from build123d import *

# Parameters (mm, degrees)
BOSS_EXTRUDE1_DEPTH = 70
SKETCH2_R           = 5
CUT_EXTRUDE1_DEPTH  = 816
SKETCH3_R           = 10
CUT_EXTRUDE2_DEPTH  = 143
FILLET1_R           = 4


with BuildPart() as part:
    # Sketch1 → Boss-Extrude1 (new body)
    with BuildSketch(Plane.XY):
        with BuildLine():
            Line((-110, 0), (90, 0))
            ThreePointArc((90, 0), (266.776695297, -73.223304703), (340, -250))
            Line((340, -250), (340, -350))
            Line((340, -350), (350, -350))
            Line((350, -350), (350, -240))
            ThreePointArc((350, -240), (276.776695297, -63.223304703), (100, 10))
            Line((100, 10), (-120, 10))
            ThreePointArc((-120, 10), (-296.776695297, -63.223304703), (-370, -240))
            Line((-370, -240), (-370, -350))
            Line((-370, -350), (-360, -350))
            Line((-360, -350), (-360, -250))
            ThreePointArc((-360, -250), (-286.776695297, -73.223304703), (-110, 0))
        make_face()
    extrude(amount=BOSS_EXTRUDE1_DEPTH)

    # Sketch2 → Cut-Extrude1 (cut)
    with BuildSketch(Plane(origin=(350, 0, 0), x_dir=(0, 0, -1), z_dir=(1, 0, 0))):
        with Locations((-36.389856075, -325)):
            Circle(SKETCH2_R)
    extrude(amount=-CUT_EXTRUDE1_DEPTH, mode=Mode.SUBTRACT)

    # Sketch3 → Cut-Extrude2 (cut)
    with BuildSketch(Plane(origin=(0, 10, 0), x_dir=(1, 0, 0), z_dir=(0, 1, 0))):
        with Locations((-65, -35)):
            Circle(SKETCH3_R)
        with Locations((-10, -35)):
            Circle(SKETCH3_R)
        with Locations((45, -35)):
            Circle(SKETCH3_R)
    extrude(amount=-CUT_EXTRUDE2_DEPTH, mode=Mode.SUBTRACT)

    # Fillet1
    fillet1_edges = [part.edges().sort_by_distance(p)[0] for p in [
        (-296.776695297, -63.223304703, 70),
        (350, -295, 0),
        (345, -350, 0),
        (340, -300, 0),
        (266.776695297, -73.223304703, 0),
        (-10, 0, 0),
        (-286.776695297, -73.223304703, 0),
        (-370, -295, 70),
        (-360, -300, 0),
        (-365, -350, 0),
        (-370, -295, 0),
        (-296.776695297, -63.223304703, 0),
        (-10, 10, 0),
        (276.776695297, -63.223304703, 0),
        (-365, -350, 70),
        (-360, -300, 70),
        (-286.776695297, -73.223304703, 70),
        (-10, 0, 70),
        (266.776695297, -73.223304703, 70),
        (340, -300, 70),
        (345, -350, 70),
        (350, -295, 70),
        (276.776695297, -63.223304703, 70),
        (-10, 10, 70),
    ]]
    fillet(fillet1_edges, radius=FILLET1_R)


solid = part.part
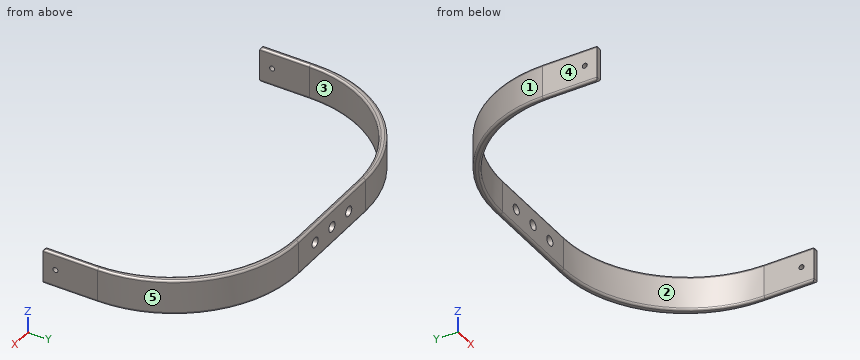
Can you work these out from the model? Positions are in its coordinate system, mm. Face numbers are marked on the shaded views. A direction names the side the tool comes from. Coordinates: 2 decimals unless noted, no trailing zeros. Write each loop counter-clockwise with the first axis right and the second up, starting at its lowest first coordinate (ties: lowest second). Pieces come first, ordered by that corner, then holes.
Q1. Imagine slicing it at B-B, the plane x = -65. List the corners of the cut face in (y, z) for me, plus the area to 3 significant figures.
Results found:
outline: (0, 4) arc R4 ccw to (4, 0) - (6, 0) arc R4 ccw to (10, 4) - (10, 25) - (0, 25) - close; (0, 45) - (10, 45) - (10, 66) arc R4 ccw to (6, 70) - (4, 70) arc R4 ccw to (0, 66) - close
area: 486 mm2
Q2. For P1, Ø10, axis at y = -105.5, z = 52, coming from the +X side; P2, Ø12, axis at x = 45, z = 35, coming from the +Y side; P3, Ø1, axis at x = 23, z = 54.5, coming from the -Y side; P4, Ø4, axis at y = -205, z = 20, coming from the -X side, each with a flat end and sliding along its axis, tell me the tip position at first contact or that it passes through.
Results found:
P1: stops at x = 313.85
P2: passes through
P3: stops at y = 0
P4: stops at x = -367.81
Q3. Please list where these lines run through material, in increasing order: L1, parallel to X at y = -313.5, z = 35; L2, parallel to Z at x = -363, y = -325; L3, parallel to X at y = -96.5, z = 34.
Results found:
L1: x = -370 to -360, 340 to 350
L2: z = 0.13 to 31.39, 41.39 to 69.87
L3: x = -324.71 to -307.33, 287.33 to 304.71
Q4. Which directions (+Z, -Z, +X, -X, +Y, -Y) give clear straight access to the entire face, cutting with the end or side of a thin tool? Please do the marked faces 1 and 2.
Results found:
face 1: +Z, -Z, -X, +Y
face 2: +Z, -Z, -Y
Q5. If we mould it in two halves opening along X, with no side actions, what happens to the marked faces 3, 4 and 5? For each: +X half, -X half, draft (parallel to the pull), parting line (faces both ways), or undercut.
Results found:
face 3: undercut
face 4: -X half
face 5: +X half
Q6. Imagine slicing it at A-A, the plane y = -282. List the corners of the cut face in (x, z) for me, plus the area to 3 significant figures.
Results found:
outline: (-370, 4) arc R4 ccw to (-366, 0) - (-364, 0) arc R4 ccw to (-360, 4) - (-360, 66) arc R4 ccw to (-364, 70) - (-366, 70) arc R4 ccw to (-370, 66) - close; (340, 4) arc R4 ccw to (344, 0) - (346, 0) arc R4 ccw to (350, 4) - (350, 66) arc R4 ccw to (346, 70) - (344, 70) arc R4 ccw to (340, 66) - close
area: 1,370 mm2
